Build history of the part. All positions in model axes, mm. A direction names the side the tool comes from. Round coordinates to 2 decimals unless told otherwise and drop trailing zeros. Write each loop counter-clockwise with the first axis right and the second up, starting at its lowest first coordinate (ties: lowest second). Pieces come first, ordered by that corner, then holes. Notation, with made-up numbers: (45.5, 30) - (57.5, 30) arc R31 cw to (57.5, 67) - close; hole circle Ø3 at (13, 3). An arc over 180 degrees is marked (long way). Write each question's results on one line, items separated by ' | '.
from build123d import *

# Parameters (mm, degrees)
SKETCH_2_W          = 32.183544672
SKETCH_2_H          = 26
EXTRUDE_1_DEPTH     = 2
FILLET_1_R          = 2
SKETCH_5_W          = 6
SKETCH_5_H          = 2
EXTRUDE_2_DEPTH     = 2.5
FILLET_2_R          = 2
SKETCH_6_R          = 1
CUT_EXTRUDE_3_DEPTH = 4
CUT_EXTRUDE_3_TAPER = 2
SKETCH_7_R          = 1
CUT_EXTRUDE_4_DEPTH = 4
CUT_EXTRUDE_4_TAPER = 2
SKETCH_8_W          = 4.5
SKETCH_8_H          = 2
EXTRUDE_3_DEPTH     = 2
SKETCH_10_W         = 2.4
SKETCH_10_H         = 1.4
EXTRUDE_4_DEPTH     = 2
EXTRUDE_4_2_DEPTH   = 2
SKETCH_11_W         = 8.5
SKETCH_11_H         = 2
EXTRUDE_5_DEPTH     = 2.5
CHAMFER_1_SIZE      = 2
CHAMFER_2_SIZE      = 1


with BuildPart() as part:
    # Sketch 2 → Extrude 1 (new body)
    with BuildSketch(Plane.XY):
        with Locations((-0.901029093, -19.434236018)):
            Rectangle(SKETCH_2_W, SKETCH_2_H)
    extrude(amount=EXTRUDE_1_DEPTH)

    # Fillet 1
    fillet_1_edges = [part.edges().sort_by_distance(p)[0] for p in [
        (15.190743243, -32.434236018, 1),
        (15.190743243, -6.434236018, 1),
    ]]
    fillet(fillet_1_edges, radius=FILLET_1_R)

    # Sketch 5 → Extrude 2 (add)
    with BuildSketch(Plane(origin=(0, 0, 0), x_dir=(-1, 0, 0), z_dir=(0, 0, -1))):
        with Locations((-10.007198571, -7.434236018)):
            Rectangle(SKETCH_5_W, SKETCH_5_H)
        with Locations((-10.007198571, -31.434236018)):
            Rectangle(SKETCH_5_W, SKETCH_5_H)
    extrude(amount=EXTRUDE_2_DEPTH)

    # Fillet 2
    fillet_2_edges = [part.edges().sort_by_distance(p)[0] for p in [
        (13.007198571, -7.434236018, -2.5),
        (7.007198571, -7.434236018, -2.5),
        (13.007198571, -31.434236018, -2.5),
        (7.007198571, -31.434236018, -2.5),
    ]]
    fillet(fillet_2_edges, radius=FILLET_2_R)

    # Sketch 6 → Cut-Extrude 3 (cut)
    with BuildSketch(Plane.XZ.offset(32.434236018)):
        with Locations((10.190743244, -0.5)):
            Circle(SKETCH_6_R)
    extrude(amount=-CUT_EXTRUDE_3_DEPTH, taper=CUT_EXTRUDE_3_TAPER, mode=Mode.SUBTRACT)

    # Sketch 7 → Cut-Extrude 4 (cut)
    with BuildSketch(Plane(origin=(0, -6.434236018, 0), x_dir=(1, 0, 0), z_dir=(0, 1, 0))):
        with Locations((10.190743243, 0.5)):
            Circle(SKETCH_7_R)
    extrude(amount=-CUT_EXTRUDE_4_DEPTH, taper=CUT_EXTRUDE_4_TAPER, mode=Mode.SUBTRACT)

    # Sketch 8 → Extrude 3 (add)
    with BuildSketch(Plane(origin=(0, 0, 0), x_dir=(-1, 0, 0), z_dir=(0, 0, -1))):
        with Locations((19.242801429, -12.484236018)):
            Rectangle(SKETCH_8_W, SKETCH_8_H)
        with Locations((19.242801429, -26.484236018)):
            Rectangle(SKETCH_8_W, SKETCH_8_H)
    extrude(amount=-EXTRUDE_3_DEPTH)



with BuildPart() as body_2:
    # Sketch 10 → Extrude 4 (new body)
    with BuildSketch(Plane(origin=(0, 0, 0), x_dir=(-1, 0, 0), z_dir=(0, 0, -1))):
        with Locations((20.292801429, -14.184236018)):
            Rectangle(SKETCH_10_W, SKETCH_10_H)
    extrude(amount=-EXTRUDE_4_DEPTH)


with BuildPart() as body_3:
    # Sketch 10 → Extrude 4 2 (new body)
    with BuildSketch(Plane(origin=(0, 0, 0), x_dir=(-1, 0, 0), z_dir=(0, 0, -1))):
        with Locations((20.292801429, -28.184236018)):
            Rectangle(SKETCH_10_W, SKETCH_10_H)
    extrude(amount=-EXTRUDE_4_2_DEPTH)


with BuildPart() as part_1:
    add(part.part)

    add(body_2.part)  # Extrude 5 merges body 2

    add(body_3.part)  # Extrude 5 merges body 3
    # Sketch 11 → Extrude 5 (add)
    with BuildSketch(Plane(origin=(0, 0, 0), x_dir=(-1, 0, 0), z_dir=(0, 0, -1))):
        with Locations((17.242801429, -12.484236018)):
            Rectangle(SKETCH_11_W, SKETCH_11_H)
        with Locations((17.242801429, -26.484236018)):
            Rectangle(SKETCH_11_W, SKETCH_11_H)
    extrude(amount=EXTRUDE_5_DEPTH)

    # Chamfer 1
    chamfer_1_edges = [part_1.edges().sort_by_distance(p)[0] for p in [
        (-21.492801429, -12.484236018, -2.5),
        (-12.992801429, -12.484236018, -2.5),
        (-21.492801429, -26.484236018, -2.5),
        (-12.992801429, -26.484236018, -2.5),
    ]]
    chamfer(chamfer_1_edges, length=CHAMFER_1_SIZE)

    # Chamfer 2
    chamfer_2_edges = [part_1.edges().sort_by_distance(p)[0] for p in [
        (-21.492801429, -14.884236018, 1),
        (-21.492801429, -28.884236018, 1),
    ]]
    chamfer(chamfer_2_edges, length=CHAMFER_2_SIZE)


solid = part_1.part
(1) Flat gauge pins, fed straight in: pin 1 Ø0.6 at (y, z) = (-17, 1.5) entering from -X; pin 2 Ø1.4 at (x, z) = (-16, -1) entering from +Y; pin 3 Ø0.7 at (x, y) = (-20, -14) entering from -Z. Where does each tip first touch, or does it go through?
Worked answers:
pin 1: stops at x = -16.99 | pin 2: stops at y = -11.48 | pin 3: stops at z = 0
(2) Slice it at A-A, the plane z = 1.1. Write the cut outline in (x, y).
Worked answers:
outline: (-21.49, -27.88) - (-20.49, -28.88) - (-19.09, -28.88) - (-19.09, -27.48) - (-16.99, -27.48) - (-16.99, -32.43) - (13.19, -32.43) arc R2 ccw to (15.19, -30.43) - (15.19, -8.43) arc R2 ccw to (13.19, -6.43) - (-16.99, -6.43) - (-16.99, -11.48) - (-21.49, -11.48) - (-21.49, -13.88) - (-20.49, -14.88) - (-19.09, -14.88) - (-19.09, -13.48) - (-16.99, -13.48) - (-16.99, -25.48) - (-21.49, -25.48) - close
(3) Tool access for faces 1 (the flat face through (-18, -25.484, 0)), 2 (the flat face through (-20.986, -14.391, 0.986)), 3 (the flat face through (-13.98, -26.5, -1.49)): list every direction of +Z, -Z, +X, -X, +Y, -Y with a clear straight run to the whole face (end or side of a thin tool).
Worked answers:
face 1: -Z, -X | face 2: +Z, -Z, -X | face 3: -Z, +X, +Y, -Y
(4) Slice it at C-C, the plane y = -18.75. Write the cut outline in (x, z).
Worked answers:
outline: (-16.99, 0) - (15.19, 0) - (15.19, 2) - (-16.99, 2) - close
(5) Slice it at D-D, the plane x = 8.5. Write the cut outline in (y, z).
Worked answers:
outline: (-32.43, -2.43) - (-30.43, -2.43) - (-30.43, 0) - (-8.43, 0) - (-8.43, -2.43) - (-6.43, -2.43) - (-6.43, 2) - (-32.43, 2) - close
(6) Two-plate mould, pull along Y, no slides. Class faces 4 (the conical face through (9.986, -8.018, 0.422)), 5 (the flat face through (10, -30.434, -2)), 6 (the cylindrical face through (7.58, -7.42, -1.9)): released by +Y, released by -Y, zero draft, split by the parting line, or undercut.
Worked answers:
face 4: released by +Y | face 5: undercut | face 6: zero draft
(7) Slice it at B-B, the plane x = -2.5. Write the cut outline in (y, z).
Worked answers:
outline: (-32.43, 0) - (-6.43, 0) - (-6.43, 2) - (-32.43, 2) - close
(8) Drill centre lines: probe 1 along X at (y, z) = (-13.75, 0.95); probe 2 along Y at (x, z) = (-14.5, -0.5); probe 3 along Z at (x, y) = (-2, -15). Where is each one in solid material? Low to high. Write a range as [from, to].
Worked answers:
probe 1: x = [-21.49, -19.09], [-16.99, 15.19] | probe 2: y = [-27.48, -25.48], [-13.48, -11.48] | probe 3: z = [0, 2]
